Autodesk Inventor part; units mm, degrees
ref_plane "YZ Plane" through (0, 0, 0) normal (1, 0, 0) x (0, 1, 0)
ref_plane "XZ Plane" through (0, 0, 0) normal (0, 1, 0) x (-1, 0, 0)
ref_plane "XY Plane" through (0, 0, 0) normal (0, 0, 1) x (1, 0, 0)
sketch "Skizze2" plane through (0, 0, 0) normal (0, 0, 1) x (1, 0, 0)
  line L0 (-30.3771, 139.6504) -> (269.6229, 139.6504)
  line L1 (269.6229, 139.6504) -> (269.6229, -10.3496)
  line L2 (269.6229, -10.3496) -> (-30.3771, -10.3496)
  line L3 (-30.3771, -10.3496) -> (-30.3771, 139.6504)
  point P0 (0, 0)
  dimension "d4" = 300
  dimension "d5" = 150
extrude "Extrusion2" add sketch "Skizze2" along normal blind 30
sketch "Skizze3" plane through (0, 0, 30) normal (0, 0, 1) x (1, 0, 0)
  line L0 (-30.3771, 139.6504) -> (-30.3771, -10.3496)
  line L1 (269.6229, -10.3496) -> (269.6229, 139.6504)
  line L2 (-30.3771, 84.6504) -> (269.6229, 84.6504)
  line L3 (269.6229, 84.6504) -> (269.6229, 44.6504)
  line L4 (269.6229, 44.6504) -> (-30.3771, 44.6504)
  line L5 (-30.3771, 44.6504) -> (-30.3771, 84.6504)
  line L6 (269.6229, 139.6504) -> (-30.3771, 139.6504)
  point P0 (0, 0)
  dimension "d8" = 40
  dimension "d9" = 55
extrude "Extrusion3" cut sketch "Skizze3" against normal blind 3 contours L2 L1 L4 L0
sketch "Skizze5" plane through (0, 0, 30) normal (0, 0, 1) x (1, 0, 0)
  line L0 (-30.3771, -10.3496) -> (269.6229, -10.3496)
  line L1 (269.6229, 139.6504) -> (-30.3771, 139.6504)
  line L2 (99.6229, -10.3496) -> (139.6229, -10.3496)
  line L3 (139.6229, -10.3496) -> (139.6229, 139.6504)
  line L4 (139.6229, 139.6504) -> (99.6229, 139.6504)
  line L5 (99.6229, 139.6504) -> (99.6229, -10.3496)
  line L6 (-30.3771, 139.6504) -> (-30.3771, 84.6504)
  point P0 (0, 0)
  dimension "d15" = 40
  dimension "d16" = 130
extrude "Extrusion4" cut sketch "Skizze5" against normal blind 3
sketch "Skizze6" plane through (0, 0, 30) normal (0, 0, 1) x (1, 0, 0)
  line L0 (-30.3771, 139.6504) -> (-30.3771, -10.3496)
  line L1 (-30.3771, 139.6504) -> (79.6229, 139.6504)
  line L2 (79.6229, 139.6504) -> (79.6229, 104.6504)
  line L3 (79.6229, 104.6504) -> (-30.3771, 104.6504)
  line L4 (-30.3771, 104.6504) -> (-30.3771, 139.6504)
  line L5 (269.6229, 139.6504) -> (139.6229, 139.6504)
  line L6 (269.6229, 139.6504) -> (159.6229, 139.6504)
  line L7 (159.6229, 139.6504) -> (159.6229, 104.6504)
  line L8 (159.6229, 104.6504) -> (269.6229, 104.6504)
  line L9 (269.6229, 104.6504) -> (269.6229, 139.6504)
  line L10 (269.6229, -10.3496) -> (269.6229, 44.6504)
  line L11 (269.6229, -10.3496) -> (159.6229, -10.3496)
  line L12 (159.6229, -10.3496) -> (159.6229, 24.6504)
  line L13 (159.6229, 24.6504) -> (269.6229, 24.6504)
  line L14 (269.6229, 24.6504) -> (269.6229, -10.3496)
  line L15 (-30.3771, -10.3496) -> (79.6229, -10.3496)
  line L16 (79.6229, -10.3496) -> (79.6229, 24.6504)
  line L17 (79.6229, 24.6504) -> (-30.3771, 24.6504)
  line L18 (-30.3771, 24.6504) -> (-30.3771, -10.3496)
  point P0 (0, 0)
  dimension "d19" = 110
  dimension "d20" = 35
  dimension "d21" = 110
  dimension "d22" = 35
  dimension "d23" = 110
  dimension "d24" = 35
  dimension "d25" = 110
  dimension "d26" = 35
extrude "Extrusion5" add sketch "Skizze6" along normal blind 100 contours L1 L2 L3 L0
sketch "Skizze7" plane through (0, 0, 0) normal (0, 0, -1) x (-1, 0, 0)
  line L0 (20.3771, -0.3496) -> (-259.6229, -0.3496)
  line L1 (-259.6229, -0.3496) -> (-259.6229, 129.6504)
  line L2 (-259.6229, 129.6504) -> (20.3771, 129.6504)
  line L3 (20.3771, 129.6504) -> (20.3771, -0.3496)
  line L4 (30.3771, -10.3496) -> (-269.6229, -10.3496)
  line L5 (30.3771, 139.6504) -> (30.3771, -10.3496)
  line L6 (-234.6229, -10.3496) -> (-244.6229, -10.3496)
  line L7 (-244.6229, -10.3496) -> (-244.6229, -0.3496)
  line L8 (-244.6229, -0.3496) -> (-234.6229, -0.3496)
  line L9 (-234.6229, -0.3496) -> (-234.6229, -10.3496)
  line L10 (-269.6229, -10.3496) -> (-269.6229, 139.6504)
  point P0 (0, 0)
  point P1 (-239.6229, -10.3496)
  point P2 (-244.6229, -5.3496)
  dimension "d29" = 280
  dimension "d30" = 130
  dimension "d31" = 10
  dimension "d32" = 10
  dimension "d33" = 10
  dimension "d34" = 10
  dimension "d36" = 0
  dimension "d37" = 25
extrude "Extrusion6" cut sketch "Skizze7" against normal blind 20
sketch "Skizze8" plane through (0, 0, 30) normal (0, 0, 1) x (1, 0, 0)
  circle A0 centre (89.6229, 94.6504) radius 5
  line L0 (-30.3771, 84.6504) -> (99.6229, 84.6504)
  line L1 (99.6229, 84.6504) -> (99.6229, 139.6504)
  circle A1 centre (89.6229, 34.6504) radius 5
  line L2 (99.6229, 44.6504) -> (-30.3771, 44.6504)
  line L3 (99.6229, -10.3496) -> (99.6229, 44.6504)
  circle A2 centre (149.6229, 34.6504) radius 5
  line L4 (139.6229, 44.6504) -> (139.6229, -10.3496)
  circle A3 centre (149.6229, 94.6504) radius 5
  line L5 (139.6229, 139.6504) -> (139.6229, 84.6504)
  point P0 (0, 0)
  dimension "d40" = 10
  dimension "d41" = 10
  dimension "d42" = 10
  dimension "d43" = 10
  dimension "d44" = 10
  dimension "d45" = 10
  dimension "d46" = 10
  dimension "d47" = 10
  dimension "d48" = 10
  dimension "d49" = 10
extrude "Extrusion7" cut sketch "Skizze8" against normal through all
extrude "Extrusion8" add sketch "Skizze6" along normal blind 80 contours L9 L8 L7 L5
extrude "Extrusion9" add sketch "Skizze6" along normal blind 90 contours L17 L16 L15 L0
extrude "Extrusion10" add sketch "Skizze6" along normal blind 95 contours L11 L12 L13 L10
sketch "Skizze12" plane through (0, 0, 20) normal (0, 0, -1) x (-1, 0, 0)
  line L0 (-259.6229, 129.6504) -> (20.3771, 129.6504)
  line L1 (20.3771, 129.6504) -> (-69.6229, 129.6504)
  line L2 (-69.6229, 129.6504) -> (-69.6229, 114.6504)
  line L3 (-69.6229, 114.6504) -> (20.3771, 114.6504)
  line L4 (20.3771, 114.6504) -> (20.3771, 129.6504)
  line L5 (20.3771, -0.3496) -> (-234.6229, -0.3496)
  line L6 (20.3771, -0.3496) -> (-69.6229, -0.3496)
  line L7 (-69.6229, -0.3496) -> (-69.6229, 14.6504)
  line L8 (-69.6229, 14.6504) -> (20.3771, 14.6504)
  line L9 (20.3771, 14.6504) -> (20.3771, -0.3496)
  line L10 (-259.6229, 129.6504) -> (-169.6229, 129.6504)
  line L11 (-169.6229, 129.6504) -> (-169.6229, 114.6504)
  line L12 (-169.6229, 114.6504) -> (-259.6229, 114.6504)
  line L13 (-259.6229, 114.6504) -> (-259.6229, 129.6504)
  line L14 (-259.6229, -0.3496) -> (-169.6229, -0.3496)
  line L15 (-169.6229, -0.3496) -> (-169.6229, 14.6504)
  line L16 (-169.6229, 14.6504) -> (-259.6229, 14.6504)
  line L17 (-259.6229, 14.6504) -> (-259.6229, -0.3496)
  point P0 (0, 0)
  dimension "d58" = 90
  dimension "d59" = 15
  dimension "d60" = 90
  dimension "d61" = 15
  dimension "d62" = 90
  dimension "d63" = 15
  dimension "d64" = 90
  dimension "d65" = 15
extrude "Extrusion11" cut sketch "Skizze12" against normal blind 70
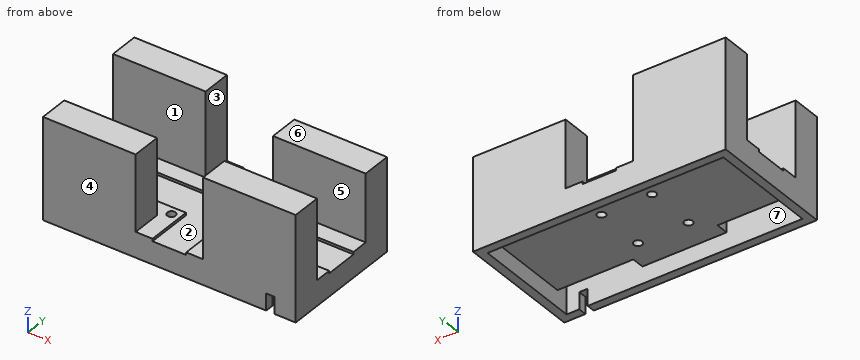
Can you work these out from the model? Positions are in its coordinate system, mm. Face numbers are marked on the shaded views. A direction names the side the tool comes from. Coordinates: 2 decimals unless noted, no trailing zeros. Loops run counter-clockwise (first coordinate to the right, second up) from the corner with the lowest first, then second, coordinate; pieces in that order, holes last. Notation, with made-up numbers: (69, -24) - (96, -24) arc R23 cw to (96, 0) - close; hole circle Ø4 at (19.25, 79). An arc over 180 degrees is marked (long way). Put each result on its own line as item: value. Start each with the question number.
Item 1: Suppose I cut it at C-C (z = 116.5). Please give me the cut outline in (x, y), and give its area (4 significant figures).
Item 2: Suppose I cut it at D-D (x = 28). Please give me the cut outline in (y, z).
Item 3: If we mould it in two halves opening along Y, with no side actions, what happens to the marked faces 1, 2, 3 and 4? For each: +Y half, -Y half, draft (parallel to the pull), parting line (faces both ways), or undercut.
Item 4: Which directions (+Z, -Z, +X, -X, +Y, -Y) give clear straight access to the entire face, cutting with the end or side of a thin tool? Please do the marked faces 5, 6 and 7.
Item 5: Suppose I cut it at B-B (y = 57). Please give me the cut outline in (x, z), and give its area (3 significant figures).
Item 6: For pin 1 (17.5 mm diameter, centred on x = 220.5, y = 0, fed in from +Z); pin 2 (16.5 mm diameter, centred on x = 18.5, y = 124.5, fed in from -Z); pin 3 (10 mm diameter, centred on x = 162, y = 112, fed in from +Z); pin 4 (8 mm diameter, centred on x = 166, y = 54, fed in from +Z), each with a flat end and sliding along its axis, tell me the tip position at first contact or that it passes through.
Item 7: Suppose I cut it at A-A (z = 71). State how many separate pieces and enclosed holes the cut face has, and give its area (3 significant figures).
Item 8: If I drill on line 1 along X through (y, z) = (6, 41.5); line 2 along Y through (x, z) = (-2, 68); line 3 along Y through (x, z) = (14, 29), over which ranges is the centre line in solid material (lowest first)?
Here are the results:
1. outline: (-30.38, -10.35) - (79.62, -10.35) - (79.62, 24.65) - (-30.38, 24.65) - close; (-30.38, 104.65) - (79.62, 104.65) - (79.62, 139.65) - (-30.38, 139.65) - close; (159.62, -10.35) - (269.62, -10.35) - (269.62, 24.65) - (159.62, 24.65) - close
1. area: 11,550 mm²
2. outline: (-10.35, 0) - (-0.35, 0) - (-0.35, 90) - (14.65, 90) - (14.65, 20) - (114.65, 20) - (114.65, 90) - (129.65, 90) - (129.65, 0) - (139.65, 0) - (139.65, 130) - (104.65, 130) - (104.65, 30) - (84.65, 30) - (84.65, 27) - (44.65, 27) - (44.65, 30) - (24.65, 30) - (24.65, 120) - (-10.35, 120) - close
3. face 1: undercut
3. face 2: undercut
3. face 3: draft
3. face 4: -Y half
4. face 5: +Z, +X, -X
4. face 6: +Z, +X, +Y
4. face 7: -Z
5. outline: (-30.38, 0) - (-20.38, 0) - (-20.38, 20) - (259.62, 20) - (259.62, 0) - (269.62, 0) - (269.62, 27) - (-30.38, 27) - close
5. area: 2,500 mm²
6. pin 1: z = 125
6. pin 2: z = 0
6. pin 3: z = 110
6. pin 4: z = 27
7. separate pieces: 4
7. enclosed holes: 4
7. area: 10,000 mm²
8. line 1: -30.38 to -20.38, 69.62 to 79.62, 159.62 to 169.62, 259.62 to 269.62
8. line 2: -10.35 to -0.35, 14.65 to 24.65, 104.65 to 114.65, 129.65 to 139.65
8. line 3: -10.35 to -0.35, 14.65 to 44.65, 84.65 to 114.65, 129.65 to 139.65
